Design review of the part built by this model. Coordinates are the model's own, in mm. A direction names the side the tool comes from. Coordinates: 2 decimals unless noted, no trailing zeros. Loops run counter-clockwise (first coordinate to the right, second up) from the corner with the lowest first, then second, coordinate; pieces in that order, holes last. Notation, with made-up numbers: (11, -3) - (57, -3) arc R17 ccw to (57, 11) - close; hole circle Ø5 at (53, 21.25). An arc over 180 degrees is marked (long way). Return JSON: item names as keys, results as strings. Group by question number.
from build123d import *

# Parameters (mm, degrees)
SKETCH001_W     = 299
SKETCH001_H     = 109
SKETCH001_W_2   = 287
SKETCH001_H_2   = 97
PAD_DEPTH       = 12
SKETCH002_W     = 295
SKETCH002_H     = 105
POCKET_DEPTH    = 3
SKETCH003_W     = 80
SKETCH003_H     = 4
POCKET001_DEPTH = 4
SKETCH004_W     = 4
SKETCH004_H     = 32.5
POCKET002_DEPTH = 4


with BuildPart() as part:
    # Sketch001 → Pad (new body)
    with BuildSketch(Plane.XY):
        Rectangle(SKETCH001_W, SKETCH001_H)
        Rectangle(SKETCH001_W_2, SKETCH001_H_2, mode=Mode.SUBTRACT)
    extrude(amount=PAD_DEPTH)

    # Sketch002 (on Face9 of Pad) → Pocket (cut)
    with BuildSketch(Plane(origin=(0, 0, 0), x_dir=(1, 0, 0), z_dir=(0, 0, -1))):
        Rectangle(SKETCH002_W, SKETCH002_H)
    extrude(amount=-POCKET_DEPTH, mode=Mode.SUBTRACT)

    # Sketch003 (on Face15 of Pocket) → Pocket001 (cut)
    with BuildSketch(Plane(origin=(0, 0, 3), x_dir=(1, 0, 0), z_dir=(0, 0, -1))):
        with Locations((-95, 50.5)):
            Rectangle(SKETCH003_W, SKETCH003_H)
        with Locations((0, 50.5)):
            Rectangle(SKETCH003_W, SKETCH003_H)
        with Locations((95, 50.5)):
            Rectangle(SKETCH003_W, SKETCH003_H)
        with Locations((-95, -50.5)):
            Rectangle(SKETCH003_W, SKETCH003_H)
        with Locations((0, -50.5)):
            Rectangle(SKETCH003_W, SKETCH003_H)
        with Locations((95, -50.5)):
            Rectangle(SKETCH003_W, SKETCH003_H)
    extrude(amount=-POCKET001_DEPTH, mode=Mode.SUBTRACT)

    # Sketch004 (on Face15 of Pocket001) → Pocket002 (cut)
    with BuildSketch(Plane(origin=(0, 0, 3), x_dir=(1, 0, 0), z_dir=(0, 0, -1))):
        with Locations((145.5, 23.75)):
            Rectangle(SKETCH004_W, SKETCH004_H)
        with Locations((145.5, -23.75)):
            Rectangle(SKETCH004_W, SKETCH004_H)
        with Locations((-145.5, 23.75)):
            Rectangle(SKETCH004_W, SKETCH004_H)
        with Locations((-145.5, -23.75)):
            Rectangle(SKETCH004_W, SKETCH004_H)
    extrude(amount=-POCKET002_DEPTH, mode=Mode.SUBTRACT)


solid = part.part
Item 1: Add section A-A (x = -82). State the section outline as (y, z) points.
Item 2: Add section B-B (y = 26.5). State the section outline as (x, z) points, then the cut area to 3 significant figures.
Item 3: Draft analysis for pull direction X (two halves, no side actions). For faces 4 (the face through (-1, 53, 0)), 5 (the face through (143, 49, 3)), 6 (the face through (149.5, -1, 6)), 7 (the face through (-149.5, -1, 6)), state which applies: pulls with the +X half, pulls with the -X half, needs draft (parallel to the pull), parting line crosses it, or undercut.
Item 4: For faces 1 (the face through (-143.5, -1, 8)), 2 (the face through (-2, 52.5, 3)), 3 (the face through (-45, 49, 12)), list the 3-axis set-ups (+Z, -Z, +X, -X, +Y, -Y) from which the entire face can be reached by the end or side of a thin tool; tool diameter is ignored.
Item 5: To check wall thickness, follow line 1 (X direction, y = -5, z = 1.25); line 2 (X direction, y = 48, z = 7); line 3 (Y direction, x = -64, z = 8). State the ranges of each line that lie inside material, in increasing order. Write a range as from..to.
Item 6: Add section C-C (z = 9). State the section outline as (x, y) points, then the cut area to 3 significant figures.
Item 7: For P1, Ø1.2, axis at x = 146, y = 3.5, coming from the -Z side; P2, Ø2, axis at x = 75.5, y = 51, coming from the -Z side, all flat-tipped, find the tip position at first contact; note any pin that passes through.
Answers below:
{
 "1": {"outline": "(-54.5, 0) - (-52.5, 0) - (-52.5, 7) - (-48.5, 7) - (-48.5, 12) - (-54.5, 12) - close; (48.5, 7) - (52.5, 7) - (52.5, 0) - (54.5, 0) - (54.5, 12) - (48.5, 12) - close"},
 "2": {"outline": "(-149.5, 0) - (-147.5, 0) - (-147.5, 7) - (-143.5, 7) - (-143.5, 12) - (-149.5, 12) - close; (143.5, 7) - (147.5, 7) - (147.5, 0) - (149.5, 0) - (149.5, 12) - (143.5, 12) - close", "area": "88.0 mm^2"},
 "3": {"face 4": "needs draft", "face 5": "undercut", "face 6": "pulls with the +X half", "face 7": "pulls with the -X half"},
 "4": {"face 1": "+Z, -Z", "face 2": "-Z", "face 3": "+Z, +X, -X, +Y, -Y"},
 "5": {"line 1": "x = -149.5..-147.5, 147.5..149.5", "line 2": "x = -149.5..-143.5, 143.5..149.5", "line 3": "y = -54.5..-48.5, 48.5..54.5"},
 "6": {"outline": "(-149.5, -54.5) - (149.5, -54.5) - (149.5, 54.5) - (-149.5, 54.5) - close; hole (-143.5, -48.5) - (143.5, -48.5) - (143.5, 48.5) - (-143.5, 48.5) - close", "area": "4,750 mm^2"},
 "7": {"P1": "stops at z = 3", "P2": "stops at z = 7"}
}
